Part model, mm, in its own coordinate system. A direction names the side the tool comes from. Round coordinates to 2 decimals unless told otherwise and drop trailing zeros. Write each loop counter-clockwise with the first axis right and the second up, starting at its lowest first coordinate (ties: lowest second). Pieces come first, ordered by that corner, then holes. Notation, with made-up numbers: M -34,29 L 18,29 A24 ccw 18,45 Z; hole C 4.25,0 d1. An arc over 180 degrees is marked long. Use a Markdown table: item, result. Add a question column.
1) Slice it at A-A on z = 105. Give the number of separate pieces and of enclosed holes in the cut face, plus the area to 3 significant figures.
2) Slice it at B-B on z = 36. Write the cut outline in (x, y), plus the area to 3 significant figures.
3) Drop flat-ended pins along their axis: P1, Ø11.5, axis at x = 12.5, z = 15, coming from the -Y side; P2, Ø2, axis at y = 12.5, z = 75.5, coming from the -X side; P3, Ø5, axis at x = 14.5, z = 95.5, coming from the +Y side. Give the stop position or say it passes through.
4) Slice it at C-C on x = 18.5. Write the cut outline in (y, z), plus the area to 3 significant figures.
5) Which spindle directions (+Z, -Z, +X, -X, +Y, -Y) get a long thin tool onto all of the face, cutting with end or side? Do faces 1 (the face through (58, 5, 117)), 2 (the face through (48, 10, 59)), 3 (the face through (47, 8, 10)). Say none if no direction does.
6) Two-plate mould, pull along Z, no slides. Class faces 4 (the face through (45.081, 9.014, 78.794)), 5 (the face through (57, 5, 2)), 6 (the face through (25, 13, 59)): released by +Z, released by -Z, zero draft, split by the parting line, or undercut.
7) Wall check: probe 1 along Z at (x, y) = (47.5, 8.55); probe 2 along X at (y, z) = (9.4, 15); probe 3 along Z at (x, y) = (47.5, 2.25). Give the ranges that are in metal, low to high.
```python
from build123d import *

# Parameters (mm, degrees)
F1_DEPTH       = 120
F3_D           = 9
F3_DEPTH       = 10
F3_CBORE_D     = 15
F3_CBORE_DEPTH = 8
F3_TIP         = 2.7038727856
F4_SIZE        = 5
F5_SIZE        = 0.5


with BuildPart() as f1:
    # F0 (on Top) → F1 (new body)
    with BuildSketch(Plane.XY):
        Polygon((0, 10), (0, 0), (60, 0), (60, 10), (35, 10), (35, 15), (25, 15), (25, 10), align=None)
    extrude(amount=F1_DEPTH)

    # F3
    with Locations(Plane.XZ):
        with Locations((47.5, 45), (47.5, 75), (12.5, 15), (12.5, 105), (47.5, 15), (12.5, 75), (47.5, 105), (12.5, 45)):
            CounterBoreHole(F3_D / 2, F3_CBORE_D / 2, F3_CBORE_DEPTH, depth=F3_DEPTH)
            with Locations((0, 0, -(F3_DEPTH + F3_TIP / 2))):  # 118° drill point
                Cone(0, F3_D / 2, F3_TIP, mode=Mode.SUBTRACT)

    # F4
    f4_edges = [f1.edges().sort_by_distance(p)[0] for p in [
        (0, 5, 120),
        (60, 5, 120),
        (60, 5, 0),
        (0, 5, 0),
    ]]
    chamfer(f4_edges, length=F4_SIZE)

    # F5
    f5_edges = [f1.edges().sort_by_distance(p)[0] for p in [
        (35, 15, 60),
        (25, 15, 60),
        (0, 10, 60),
        (60, 10, 60),
        (35, 10, 60),
        (25, 10, 60),
    ]]
    chamfer(f5_edges, length=F5_SIZE)


solid = f1.part
```
Entries:
| question | item | result |
|---|---|---|
| 1 | separate pieces | 3 |
| 1 | enclosed holes | 0 |
| 1 | area | 374 mm^2 |
| 2 | outline | M 0,0 L 60,0 L 60,9.5 L 59.5,10 L 35.5,10 L 35,10.5 L 35,14.5 L 34.5,15 L 25.5,15 L 25,14.5 L 25,10.5 L 24.5,10 L 0.5,10 L 0,9.5 Z |
| 2 | area | 650 mm^2 |
| 3 | P1 | stops at y = 8 |
| 3 | P2 | stops at x = 25 |
| 3 | P3 | stops at y = 10 |
| 4 | outline | M 0,0 L 10,0 L 10,120 L 0,120 L 0,109.5 L 8,109.5 L 8,100.5 L 0,100.5 L 0,79.5 L 8,79.5 L 8,70.5 L 0,70.5 L 0,49.5 L 8,49.5 L 8,40.5 L 0,40.5 L 0,19.5 L 8,19.5 L 8,10.5 L 0,10.5 Z |
| 4 | area | 912 mm^2 |
| 5 | face 1 | +Z, +X, +Y, -Y |
| 5 | face 2 | +Z, -Z, +X, +Y |
| 5 | face 3 | -Y |
| 6 | face 4 | undercut |
| 6 | face 5 | released by -Z |
| 6 | face 6 | zero draft |
| 7 | probe 1 | z = 0 to 10.5, 19.5 to 40.5, 49.5 to 70.5, 79.5 to 100.5, 109.5 to 120 |
| 7 | probe 2 | x = 0 to 8, 17 to 43, 52 to 60 |
| 7 | probe 3 | z = 0 to 7.5, 22.5 to 37.5, 52.5 to 67.5, 82.5 to 97.5, 112.5 to 120 |
